Verification items for the finished model (mm, model axes). A direction names the side the tool comes from. Coordinates: 2 decimals unless noted, no trailing zeros. Write each loop counter-clockwise with the first axis right and the second up, starting at its lowest first coordinate (ties: lowest second). Pieces come first, ordered by that corner, then holes. Notation, with made-up numbers: M 87.25,48 L 105.25,48 A18 ccw 105.25,66 Z; hole C 8.25,71 d3. An arc over 180 degrees is marked long. One line per item, written item: value.
```python
from build123d import *

# Parameters (mm, degrees)
BOSS_EXTRUDE1_DEPTH = 30
SKETCH15_R          = 2.25
CUT_EXTRUDE1_DEPTH  = 31
SKETCH14_R          = 2.25
CUT_EXTRUDE2_DEPTH  = 5
CHAMFER2_SIZE       = 3
CHAMFER3_SIZE       = 2
CHAMFER4_SIZE       = 5
SKETCH14_7_R        = 4
CUT_EXTRUDE3_DEPTH  = 10


with BuildPart() as part:
    # Sketch13 → Boss-Extrude1 (new body)
    with BuildSketch(Plane.XY):
        Polygon((-26, -15.975764912), (-26, -11), (-16, -11), (-16, 10), (-11, 10), (-11, -11), (10, -11), (10, 10), (15, 10), (15, -11), (25, -11), (25, -15.975764912), align=None)
    extrude(amount=-BOSS_EXTRUDE1_DEPTH)

    # Sketch15 → Cut-Extrude1 (cut)
    with BuildSketch(Plane(origin=(15, 0, 0), x_dir=(0, 0, -1), z_dir=(1, 0, 0))):
        with Locations((5, 0)):
            Circle(SKETCH15_R)
        with Locations((25, 0)):
            Circle(SKETCH15_R)
    extrude(amount=-CUT_EXTRUDE1_DEPTH, mode=Mode.SUBTRACT)

    # Sketch14 → Cut-Extrude2 (cut)
    with BuildSketch(Plane(origin=(0, -11, 0), x_dir=(1, 0, 0), z_dir=(0, 1, 0))):
        with Locations(Location((20, 25, 0), (0, 0, 180))):
            Circle(SKETCH14_R)
        with Locations(Location((20, 5, 0), (0, 0, 180))):
            Circle(SKETCH14_R)
        with Locations(Location((-21, 5, 0), (0, 0, 180))):
            Circle(SKETCH14_R)
        with Locations(Location((-21, 25, 0), (0, 0, 180))):
            Circle(SKETCH14_R)
    extrude(amount=-CUT_EXTRUDE2_DEPTH, mode=Mode.SUBTRACT)

    # Chamfer2
    chamfer2_edges = [part.edges().sort_by_distance(p)[0] for p in [
        (-13.5, 10, 0),
        (12.5, 10, 0),
        (12.5, 10, -30),
        (-13.5, 10, -30),
    ]]
    chamfer(chamfer2_edges, length=CHAMFER2_SIZE)

    # Chamfer3
    chamfer3_edges = [part.edges().sort_by_distance(p)[0] for p in [
        (25, -13.487882456, -30),
        (25, -13.487882456, 0),
        (-26, -13.487882456, 0),
        (-26, -13.487882456, -30),
    ]]
    chamfer(chamfer3_edges, length=CHAMFER3_SIZE)

    # Chamfer4
    # the kernel refuses this chamfer: 5 mm, written as the material it adds along each edge
    with BuildSketch(Plane(origin=(-16, -11, 0), x_dir=(-0.9996219169112968, -0.027495876610586317, 0), z_dir=(0, 0, -1))) as chamfer4_piece_1_section:
        Polygon((CHAMFER4_SIZE * 0.999621916911, CHAMFER4_SIZE * 0.0274958766106), (-CHAMFER4_SIZE * 0.0274958766106, CHAMFER4_SIZE * 0.999621916911), (0, 0), align=None)
    chamfer4_piece_1 = extrude(amount=30, mode=Mode.PRIVATE)
    chamfer4_piece_1 = chamfer4_piece_1 - Plane(origin=(-21, -9.300389261, -25), x_dir=(-1, 0, 0), z_dir=(0, 1, 0)) * Cylinder(2.25, 80, mode=Mode.PRIVATE)
    chamfer4_piece_1 = chamfer4_piece_1 - Plane(origin=(-21, -9.300389261, -5), x_dir=(-1, 0, 0), z_dir=(0, 1, 0)) * Cylinder(2.25, 80, mode=Mode.PRIVATE)
    add(chamfer4_piece_1)
    with BuildSketch(Plane(origin=(15, -11, 0), x_dir=(0.9996219169112968, -0.027495876610586337, 0), z_dir=(0, 0, -1))) as chamfer4_piece_2_section:
        Polygon((CHAMFER4_SIZE * 0.999621916911, -CHAMFER4_SIZE * 0.0274958766106), (-CHAMFER4_SIZE * 0.0274958766106, -CHAMFER4_SIZE * 0.999621916911), (0, 0), align=None)
    chamfer4_piece_2 = extrude(amount=30, mode=Mode.PRIVATE)
    chamfer4_piece_2 = chamfer4_piece_2 - Plane(origin=(20, -9.300389689, -25), x_dir=(-1, 0, 0), z_dir=(0, 1, 0)) * Cylinder(2.25, 80, mode=Mode.PRIVATE)
    chamfer4_piece_2 = chamfer4_piece_2 - Plane(origin=(20, -9.300389689, -5), x_dir=(-1, 0, 0), z_dir=(0, 1, 0)) * Cylinder(2.25, 80, mode=Mode.PRIVATE)
    add(chamfer4_piece_2)

    # Sketch14<7> → Cut-Extrude3 (cut)
    with BuildSketch(Plane(origin=(0, -11, 0), x_dir=(1, 0, 0), z_dir=(0, 1, 0))):
        with Locations((20, 25)):
            Circle(SKETCH14_7_R)
        with Locations((20, 5)):
            Circle(SKETCH14_7_R)
        with Locations((-21, 5)):
            Circle(SKETCH14_7_R)
        with Locations((-21, 25)):
            Circle(SKETCH14_7_R)
    extrude(amount=CUT_EXTRUDE3_DEPTH, mode=Mode.SUBTRACT)


solid = part.part
```
Item 1: Cross-section at A-A, the plane y = -3.75. Enter the section's corners in (x, z), and give its area (3 significant figures).
The answers:
outline: M -16,-30 L -11,-30 L -11,0 L -16,0 Z; M 10,-30 L 15,-30 L 15,0 L 10,0 Z
area: 300 mm²
Item 2: Draft check along X on faces 1 (the face through (-14, 9, -28)), 2 (the face through (24, -13, -1)), 3 (the face through (18.962, -13.453, -26.996)), 4 (the face through (-11, 0, -15)). Enter one of: released by +X, released by -X, zero draft, split by the parting line, or undercut.
The answers:
face 1: zero draft
face 2: released by +X
face 3: undercut
face 4: undercut
Item 3: Cross-section at D-D, the plane x = -22.5. Enter the section's corners in (y, z).
The answers:
outline: M -15.98,-30 L -11,-30 L -11,-26.68 L -15.98,-26.68 Z; M -15.98,-23.32 L -11,-23.32 L -11,-6.68 L -15.98,-6.68 Z; M -15.98,-3.32 L -11,-3.32 L -11,0 L -15.98,0 Z
Item 4: Access from +Z, -Z, +X, -X, +Y, -Y to the whole of each face (thin tool, end or side, straight path). Record for faces 5 (the face through (15, 2, -15)), 6 (the face through (16, -9, -5)), 7 (the face through (-13.465, 0.676, -27.146)), 8 (the face through (-16, 2, -15)).
The answers:
face 5: +Z, -Z, +X, +Y
face 6: +X, +Y
face 7: +X, -X
face 8: +Z, -Z, -X, +Y
Item 5: Cross-section at C-C, the plane z = -25. Give the number of separate pieces and of enclosed holes in the cut face, and give its area (3 significant figures).
The answers:
separate pieces: 5
enclosed holes: 0
area: 383 mm²
Item 6: Go/stop test with flat-tipped pins: P1, Ø7, axis at y = 0, z = -5, coming from the +X side; P2, Ø4, axis at x = 17.5, y = -0.5, coming from the +Z side; P3, Ø6.5, axis at x = 4.5, z = -13, coming from the +Y side; P4, Ø10, axis at x = -23.5, z = -9, coming from the +Y side. Record where each tip stops, or that it passes through.
The answers:
P1: stops at x = 15
P2: passes through
P3: stops at y = -11
P4: stops at y = -8.5
Item 7: Cross-section at B-B, the plane y = 0. Enter the section's corners in (x, z).
The answers:
outline: M -16,-30 L -11,-30 L -11,-27.25 L -16,-27.25 Z; M -16,-22.75 L -11,-22.75 L -11,-7.25 L -16,-7.25 Z; M -16,-2.75 L -11,-2.75 L -11,0 L -16,0 Z; M 10,-30 L 15,-30 L 15,-27.25 L 10,-27.25 Z; M 10,-22.75 L 15,-22.75 L 15,-7.25 L 10,-7.25 Z; M 10,-2.75 L 15,-2.75 L 15,0 L 10,0 Z
Item 8: Scan lines: line 1 (X direction, y = -13.15, z = -5); line 2 (Z direction, x = -21, y = -12.65); line 3 (X direction, y = 6.25, z = -10). Record each from-to range of solid material in increasing order.
The answers:
line 1: x = -26 to -23.25, -18.75 to 17.75, 22.25 to 25
line 2: z = -30 to -27.25, -22.75 to -7.25, -2.75 to 0
line 3: x = -16 to -11, 10 to 15
